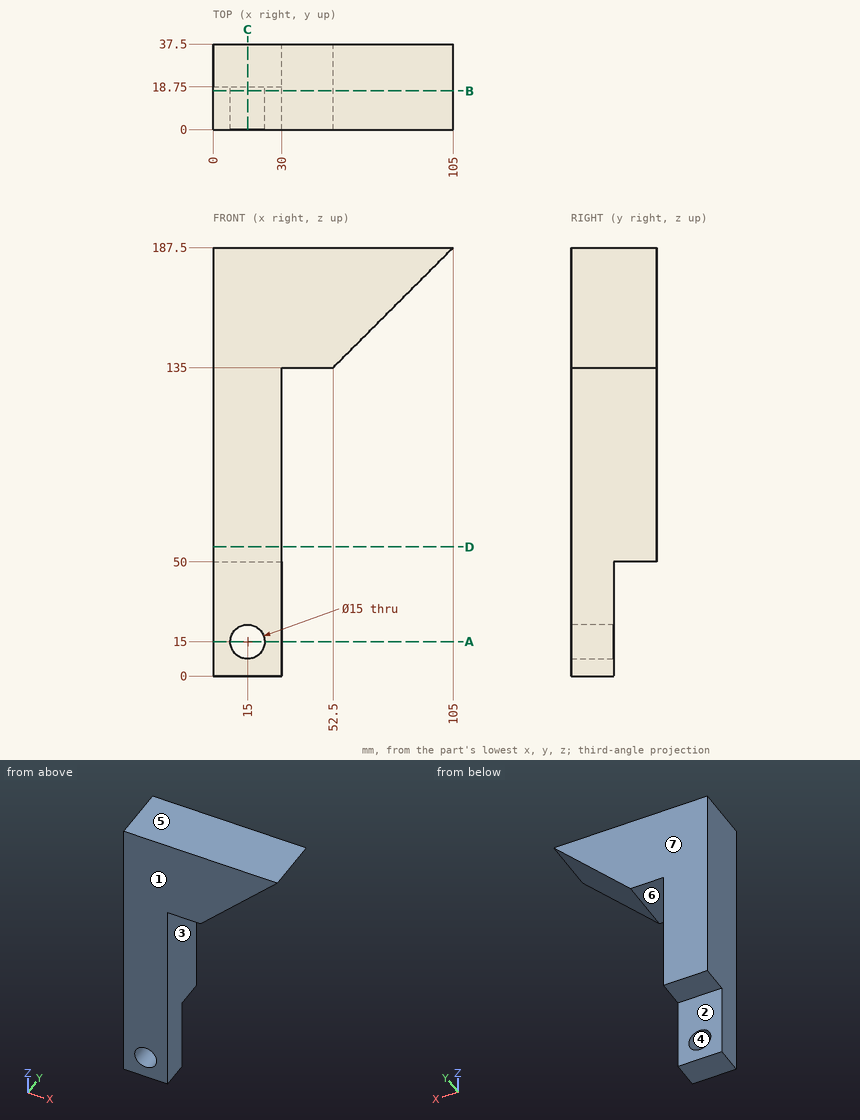
For this review, use the dimensioned drawing (mm, ordinates from the lowest corner) and the shaded views. A direction names the side the tool comes from. Coordinates: 2 decimals unless noted, no trailing zeros. Order: outer loops, then holes, each group sorted by start corner. A loop starts at its lowest first (then second) coordinate and runs counter-clockwise, first axis right, second up. Notation, with made-up numbers: M 21,25 L 75,25 A17 ccw 75,47 Z; hole C -38,29.5 d6. An arc over 180 degrees is marked long. Answer as a JSON object with one key per item and string values. Group by question number.
1) Wall thickness on L1, parallel to X at y = 4, z = 15; L2, parallel to X at y = 36, z = 120.5; L3, parallel to Y at x = 5.5, z = 48: over which ranges is each line inside the solid? List them lowest first.
2) Mouldability with a two-part tool opening along Z and no side actions: class the marked faces 4, 5, 6 and 7 as pulls with the +Z half, pulls with the -Z half, needs draft (parallel to the pull), parting line crosses it, or undercut.
3) Add section C-C, the plane x = 15. Write out the cut boundary in (y, z).
4) Add section B-B, the plane y = 17. Write out the cut boundary in (x, z), then the cut area to 3 significant figures.
5) Tool access review of the marked faces 1, 2 and 3: name each direction out of +Z, -Z, +X, -X, +Y, -Y from which nothing blocks a thin tool from reaching the whole face with its end or side.
6) For pin 1 (6 mm diameter, centred on y = 18, z = 68.5, fed in from +X); pin 2 (15 mm diameter, centred on x = 20.5, z = 37, fed in from +Y); pin 3 (11.5 mm diameter, centred on x = 46, y = 18, fed in from -Z), all flat-tipped, find the tip position at first contact; note any pin that passes through.
7) Add section D-D, the plane z = 56.5. Write out the cut boundary in (x, y), then the cut area to 4 significant figures.
8) Add section A-A, the plane z = 15. Write out the cut boundary in (x, y).
Computed values:
{
 "1": {"L1": "x = 0 to 7.5, 22.5 to 30", "L2": "x = 0 to 30", "L3": "y = 0 to 18.75"},
 "2": {"face 4": "undercut", "face 5": "pulls with the +Z half", "face 6": "pulls with the -Z half", "face 7": "needs draft"},
 "3": {"outline": "M 0,0 L 18.75,0 L 18.75,7.5 L 0,7.5 Z; M 0,22.5 L 18.75,22.5 L 18.75,50 L 37.5,50 L 37.5,187.5 L 0,187.5 Z"},
 "4": {"outline": "M 0,0 L 30,0 L 30,135 L 52.5,135 L 105,187.5 L 0,187.5 Z; hole C 15,15 d15", "area": "8,010 mm^2"},
 "5": {"face 1": "+Z, -Z, +X, -X, -Y", "face 2": "-Z, +X, -X, +Y", "face 3": "-Z, +X, +Y, -Y"},
 "6": {"pin 1": "stops at x = 30", "pin 2": "stops at y = 18.75", "pin 3": "stops at z = 135"},
 "7": {"outline": "M 0,0 L 30,0 L 30,37.5 L 0,37.5 Z", "area": "1,125 mm^2"},
 "8": {"outline": "M 0,0 L 7.5,0 L 7.5,18.75 L 0,18.75 Z; M 22.5,0 L 30,0 L 30,18.75 L 22.5,18.75 Z"}
}
